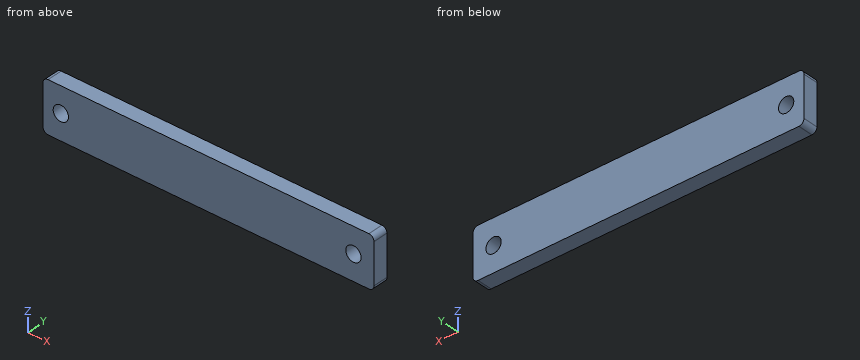
```python
from build123d import *

# Parameters (mm, degrees)
CROQUIS1_W              = 65
CROQUIS1_H              = 10
CROQUIS1_R              = 1.5
SALIENTE_EXTRUIR1_DEPTH = 3
REDONDEO1_R             = 1


with BuildPart() as part:
    # Croquis1 → Saliente-Extruir1 (new body)
    with BuildSketch(Plane(origin=(0, 0, 0), x_dir=(1, 0, 0), z_dir=(0, 1, 0))):
        with Locations((0.267609294, 1.070437174)):
            Rectangle(CROQUIS1_W, CROQUIS1_H)
        with Locations(Location((-28.732390706, 1.070437174, 0), (0, 0, 270))):
            Circle(CROQUIS1_R, mode=Mode.SUBTRACT)
        with Locations(Location((28.732390706, 1.070437174, 0), (0, 0, 90))):
            Circle(CROQUIS1_R, mode=Mode.SUBTRACT)
    extrude(amount=SALIENTE_EXTRUIR1_DEPTH)

    # Redondeo1
    redondeo1_edges = [part.edges().sort_by_distance(p)[0] for p in [
        (32.767609294, 1.5, 3.929562826),
        (-32.232390706, 1.5, 3.929562826),
        (-32.232390706, 1.5, -6.070437174),
        (32.767609294, 1.5, -6.070437174),
    ]]
    fillet(redondeo1_edges, radius=REDONDEO1_R)


solid = part.part
```
Geometry: final body of the model. Coordinates: model frame, mm. Coordinates: 2 decimals unless noted, no trailing zeros. Order: outer loops, then holes, each group sorted by start corner. A loop starts at its lowest first (then second) coordinate and runs counter-clockwise, first axis right, second up. Notation, with made-up numbers: (76, 23.25) - (113, 23.25) arc R19 ccw to (113, 47.25) - close; hole circle Ø9 at (-15.75, 50). An arc over 180 degrees is marked (long way). Return JSON: item names as keys, results as strings. Group by question number.
1. Cut plane A-A (z = -1.5). Output: boundary loops of the cut face in (x, y).
2. Material intervals for line 1 along X through (y, z) = (2, -1); line 2 along X through (y, z) = (1.6, -0.25); line 3 along X through (y, z) = (0.3, 3.5), sorted ascending. Write a range as [from, to].
3. Cut plane B-B (y = 2.55). Output: boundary loops of the cut face in (x, z).
Resolved:
{
 "1": {"outline": "(-32.23, 0) - (-30.17, 0) - (-30.17, 3) - (-32.23, 3) - close; (-27.3, 0) - (27.3, 0) - (27.3, 3) - (-27.3, 3) - close; (30.17, 0) - (32.77, 0) - (32.77, 3) - (30.17, 3) - close"},
 "2": {"line 1": "x = [-32.23, -30.23], [-27.23, 27.23], [30.23, 32.77]", "line 2": "x = [-32.23, -29.99], [-27.48, 27.48], [29.99, 32.77]", "line 3": "x = [-32.05, 32.59]"},
 "3": {"outline": "(-32.23, -5.07) arc R1 ccw to (-31.23, -6.07) - (31.77, -6.07) arc R1 ccw to (32.77, -5.07) - (32.77, 2.93) arc R1 ccw to (31.77, 3.93) - (-31.23, 3.93) arc R1 ccw to (-32.23, 2.93) - close; hole circle Ø3 at (-28.73, -1.07); hole circle Ø3 at (28.73, -1.07)"}
}
